Autodesk Inventor part; units mm, degrees
ref_plane "YZ Plane" through (0, 0, 0) normal (1, 0, 0) x (0, 1, 0)
ref_plane "XZ Plane" through (0, 0, 0) normal (0, 1, 0) x (-1, 0, 0)
ref_plane "XY Plane" through (0, 0, 0) normal (0, 0, 1) x (1, 0, 0)
sketch "Esquisse1" plane through (0, 0, 0) normal (0, 1, 0) x (-1, 0, 0)
  line L0 (8, 11.5) -> (-85, 11.5)
  line L1 (-85, 11.5) -> (-85, -11.5)
  line L2 (-85, -11.5) -> (8, -11.5)
  line L3 (8, -11.5) -> (8, 11.5)
  line L4 (0, 11.5) -> (0, -11.5) construction
  line L5 (8, 11.5) -> (42, 3)
  line L6 (42, 3) -> (42, -3)
  line L7 (42, -3) -> (8, -11.5)
  point P0 (0, 0)
  point P1 (0, 0)
  dimension "d0" = 23
  dimension "d1" = 8
  dimension "d3" = 85
  dimension "d4" = 42
  dimension "d5" = 6
extrude "Plaque1" add sketch "Esquisse1" along normal blind 3
sketch "Esquisse2" plane through (0, 3, 0) normal (0, 1, 0) x (1, 0, 0)
  line L0 (0, 0) -> (-6, 0) construction
  point P0 (0, -6)
  point P1 (6, 0)
  point P2 (0, 6)
  dimension "d9" = 360
  dimension "d11" = 6
hole "Perçage1" at (0, 3, 0) at (-6, 3, 0) at (0, 3, 6) at (6, 3, 0) at (0, 3, -6) direction (0, -1, 0) diameter 4.05 end through all counterbore diameter 5.5 counterbore depth 1
sketch "Esquisse3" plane through (0, 3, 0) normal (0, 1, 0) x (1, 0, 0)
  circle A0 centre (6, 0) radius 2.75 construction
  circle A1 centre (-6, 0) radius 2.75 construction
  circle A2 centre (0, 0) radius 2.75 construction
  circle A3 centre (0, -6) radius 2.75 construction
  circle A4 centre (0, 6) radius 2.75 construction
  line L0 (-8, -11.5) -> (-42, -3) construction
  line L1 (85, -11.5) -> (-8, -11.5) construction
  line L2 (85, 11.5) -> (85, -11.5) construction
  line L3 (-8, 11.5) -> (85, 11.5) construction
  line L4 (-42, 3) -> (-8, 11.5) construction
  line L5 (-42, -3) -> (-42, 3) construction
  line L6 (85, -11.5) -> (85, 11.5)
  line L7 (85, -4) -> (20, -11.5)
  line L8 (85, -11.5) -> (85, -4)
  line L9 (85, -11.5) -> (20, -11.5)
  line L10 (-8, -11.5) -> (85, -11.5)
  line L11 (85, 0) -> (18.7328, 0) construction
  line L12 (85, 4) -> (20, 11.5)
  line L13 (85, 11.5) -> (85, 4)
  line L14 (85, 11.5) -> (20, 11.5)
  dimension "d19" = 8
  dimension "d20" = 65
extrude "Couper1" cut sketch "Esquisse3" against normal through all
fillet "Congé1" radius 50 4 edges at (20, 1.5, 11.5) (-8, 1.5, 11.5) (20, 1.5, -11.5) (-8, 1.5, -11.5)
fillet "Congé2" radius 4 2 edges at (-42, 1.5, -3) (-42, 1.5, 3)
sketch "Esquisse4" plane through (0, 3, 0) normal (0, 1, 0) x (1, 0, 0)
  arc A0 (-38.4777, 3.8806) -> (-38.4777, -3.8806) centre (-37.5076, 0) ccw construction
  arc A1 (-13.9715, -10.0071) -> (-1.8447, -11.5) centre (-1.8447, 38.5) ccw construction
  line L0 (17.1249, -11.5) -> (-1.8447, -11.5) construction
  arc A2 (17.1249, -11.5) -> (22.8561, -11.1704) centre (17.1249, 38.5) ccw construction
  line L1 (22.8561, -11.1704) -> (85, -4) construction
  line L2 (85, 4) -> (85, -4) construction
  line L3 (85, 4) -> (22.8561, 11.1704) construction
  arc A3 (22.8561, 11.1704) -> (17.1249, 11.5) centre (17.1249, -38.5) ccw construction
  line L4 (-1.8447, 11.5) -> (17.1249, 11.5) construction
  arc A4 (-1.8447, 11.5) -> (-13.9715, 10.0071) centre (-1.8447, -38.5) ccw construction
  circle A5 centre (0, 6) radius 2.75 construction
  circle A6 centre (0, -6) radius 2.75 construction
  circle A7 centre (0, 0) radius 2.75 construction
  circle A8 centre (-6, 0) radius 2.75 construction
  circle A9 centre (6, 0) radius 2.75 construction
  line L5 (85, -4) -> (85, 4) construction
  line L6 (85, 4) -> (85, -4) construction
  line L7 (85, 0) -> (71.2936, 0) construction
  line L8 (74.9, 1.575) -> (82, 1.575)
  line L9 (82, 1.575) -> (82, -1.575)
  line L10 (82, -1.575) -> (74.9, -1.575)
  line L11 (74.9, -1.575) -> (74.9, 1.575)
  line L12 (74.9, 0) -> (82, 0) construction
  line L13 (71, 0) -> (57.2936, 0) construction
  line L14 (60.9, 1.575) -> (68, 1.575)
  line L15 (68, 1.575) -> (68, -1.575)
  line L16 (68, -1.575) -> (60.9, -1.575)
  line L17 (60.9, -1.575) -> (60.9, 1.575)
  line L18 (60.9, 0) -> (68, 0) construction
  line L19 (67, 0) -> (53.2936, 0) construction
  line L20 (42.9, -1.575) -> (42.9, 1.575)
  line L21 (50, 1.575) -> (50, -1.575)
  line L22 (50, -1.575) -> (42.9, -1.575)
  line L23 (42.9, 0) -> (50, 0) construction
  line L24 (53, 0) -> (39.2936, 0) construction
  line L25 (42.9, 1.575) -> (50, 1.575)
  line L26 (50, 0) -> (60.9, 0) construction
  circle A10 centre (55.45, 0) radius 2.05
  line L27 (-13.9715, -10.0071) -> (-38.4777, -3.8806)
  line L28 (-38.4777, 3.8806) -> (-13.9715, 10.0071)
  point P0 (61.8782, 0)
  dimension "d46" = 3.15
  dimension "d47" = 3
  dimension "d48" = 7.1
  dimension "d51" = 14
  dimension "d58" = 18
  dimension "d63" = 4.1
extrude "Couper2" cut sketch "Esquisse4" against normal blind 3
equation "\"d12\" = ollo_hole"
equation "\"d14\" = ollo_ring"
equation "\"d15\" = ollo_depth"
equation "\"d17\" = Epaisseur"
equation "\"d21\" = Epaisseur"
equation "\"d44\" = Epaisseur"
equation "\"LargeurGrugeage\" = Epaisseur"
equation "\"ProfondeurGrugeage\" = 0.5 * Epaisseur"
equation "\"TailleGrugeage\" = 4 * Epaisseur"
equation "\"RestesMinimum\" = 2 * Epaisseur"
equation "\"Rayondetransition\" = RayonPli"
equation "\"TailleRayonJacobi\" = RayonPli"
equation "\"TailleJeu\" = Epaisseur"
equation "\"d6\" = RayonPli"
properties part number "leg" material "Plastique PMMA"
Read the model definition and answer for the solid it produces. Units are mm, in the model's axes. A direction names the side the tool comes from. Round coordinates to 2 decimals unless told otherwise and drop trailing zeros. Write each loop counter-clockwise with the first axis right and the second up, starting at its lowest first coordinate (ties: lowest second). Pieces come first, ordered by that corner, then holes. Notation, with made-up numbers: (-12, 46) - (-7, 46) arc R23 cw to (-7, 58) - close; hole circle Ø4 at (60, 48). An arc over 180 degrees is marked (long way). Use CSV: the item, a comma, the result in double quotes.
Q1. A tool of negligible diameter and unlimited length cuts with its end or side. For faces 4 (the flat face through (8, 1, -11.5)), 5 (the flat face through (82, 2, 0)), 6 (the cylindrical face through (-3.315, 2.493, -0.596)), from which of +Z, -Z, +X, -X, +Y, -Y can it reach the whole face along a straight path? Write none if from no direction.
Values:
face 4,"-Z, +X, -X, +Y, -Y"
face 5,"+Y, -Y"
face 6,"+Y"
Q2. Each of these flat-tipped pins is pushed along its axis until it touches: pin 1 Ø1.5 at (x, y) = (63, 1) entering from +Z (3 decimals); pin 2 Ø4.5 at (x, z) = (6, 0) entering from +Y; pin 3 Ø1.5 at (x, y) = (45, 1.5) entering from +Z. Where does it stop, or does it pass through?
Values:
pin 1,"stops at z = 6.625"
pin 2,"stops at y = 2"
pin 3,"stops at z = 8.7"
Q3. Straight lines are drawn through the part: line 1 along Z through (x, y) = (0, 1.4) (3 decimals); line 2 along Z through (x, y) = (0, 2.7); line 3 along Z through (x, y) = (-6, 2.6). For each, find the intervals that lie inside material, in ascending order.
Values:
line 1,"z = -11.5 to -8.025, -3.975 to -2.025, 2.025 to 3.975, 8.025 to 11.5"
line 2,"z = -11.5 to -8.75, -3.25 to -2.75, 2.75 to 3.25, 8.75 to 11.5"
line 3,"z = -11.33 to -2.75, 2.75 to 11.33"
Q4. Determine the mould class of faces 1 (the flat face through (23, 0, 0)), 2 (the flat face through (64, 2, 1.575)), 3 (the cylindrical face through (-8.039, 1.521, 11.115)) for opening direction Z: +Z half, -Z half, draft (parallel to the pull), parting line (faces both ways), or undercut.
Values:
face 1,"draft"
face 2,"undercut"
face 3,"+Z half"
Q5. Find section D-D, the plane z = 6.75. Write down the section's boundary in (x, y).
Values:
outline,"(-27, 0) - (-1.88, 0) - (-1.88, 2) - (-2.65, 2) - (-2.65, 3) - (-27, 3) - close; (1.88, 0) - (61.17, 0) - (61.17, 3) - (2.65, 3) - (2.65, 2) - (1.88, 2) - close"
Q6. Find section B-B, the plane x = 76. Write down the section's boundary in (y, z) (3 decimals), then the cut area to 3 significant figures.
Values:
outline,"(0, -5.038) - (3, -5.038) - (3, -1.575) - (0, -1.575) - close; (0, 1.575) - (3, 1.575) - (3, 5.038) - (0, 5.038) - close"
area,"20.8 mm²"
Q7. Find section C-C, the plane z = 0. Count the separate pieces of the cut face and the enclosed holes in it, then the cut area to 3 significant figures.
Values:
separate pieces,"8"
enclosed holes,"0"
area,"263 mm²"
Q8. Find section A-A, the plane x = 0. Write down the section's boundary in (y, z) (3 decimals).
Values:
outline,"(0, -11.5) - (3, -11.5) - (3, -8.75) - (2, -8.75) - (2, -8.025) - (0, -8.025) - close; (0, -3.975) - (2, -3.975) - (2, -3.25) - (3, -3.25) - (3, -2.75) - (2, -2.75) - (2, -2.025) - (0, -2.025) - close; (0, 2.025) - (2, 2.025) - (2, 2.75) - (3, 2.75) - (3, 3.25) - (2, 3.25) - (2, 3.975) - (0, 3.975) - close; (0, 8.025) - (2, 8.025) - (2, 8.75) - (3, 8.75) - (3, 11.5) - (0, 11.5) - close"
